from build123d import *

# Parameters (mm, degrees)
SKETCH1_W           = 15.24
SKETCH1_H           = 15.24
BOSS_EXTRUDE1_DEPTH = 25.146
SKETCH2_R           = 5.969
CUT_EXTRUDE1_DEPTH  = 22.4536
FILLET1_R           = 7.62
CUT_EXTRUDE2_DEPTH  = 22.4536
SKETCH4_R           = 1.4605
CUT_EXTRUDE3_DEPTH  = 32.123614073
SKETCH6_W           = 16.374741922
SKETCH6_H           = 17.109502327
CUT_EXTRUDE5_DEPTH  = 20.32
SKETCH5_W           = 2.54
SKETCH5_H           = 2.54
CUT_EXTRUDE4_DEPTH  = 6.35


with BuildPart() as part:
    # Sketch1 → Boss-Extrude1 (new body)
    with BuildSketch(Plane.XY):
        with Locations((7.62, 7.62)):
            Rectangle(SKETCH1_W, SKETCH1_H)
    extrude(amount=BOSS_EXTRUDE1_DEPTH)

    # Sketch2 → Cut-Extrude1 (cut)
    with BuildSketch(Plane.XY.offset(25.146)):
        with Locations((7.62, 7.62)):
            Circle(SKETCH2_R)
    extrude(amount=-CUT_EXTRUDE1_DEPTH, mode=Mode.SUBTRACT)

    # Fillet1
    fillet1_edges = [part.edges().sort_by_distance(p)[0] for p in [
        (15.24, 15.24, 12.573),
        (0, 15.24, 12.573),
    ]]
    fillet(fillet1_edges, radius=FILLET1_R - 0.0001)  # a hair under: the kernel refuses the full size

    # Sketch3 → Cut-Extrude2 (cut)
    with BuildSketch(Plane.XY.offset(25.146)):
        with BuildLine():
            Line((11.085783791, 12.479763751), (11.085783791, 15.600426387))
            Line((11.085783791, 15.600426387), (4.154216209, 15.600426387))
            Line((4.154216209, 15.600426387), (4.154216209, 12.479763751))
            ThreePointArc((4.154216209, 12.479763751), (7.62, 13.589), (11.085783791, 12.479763751))
        make_face()
    extrude(amount=-CUT_EXTRUDE2_DEPTH, mode=Mode.SUBTRACT)

    # Sketch4 → Cut-Extrude3 (cut, through all)
    with BuildSketch(Plane.XY.offset(2.6924)):
        with Locations((7.62, 7.62)):
            Circle(SKETCH4_R)
    extrude(amount=-CUT_EXTRUDE3_DEPTH, mode=Mode.SUBTRACT)

    # Sketch6 → Cut-Extrude5 (cut)
    with BuildSketch(Plane.XY.offset(25.146)):
        with Locations((8.187370961, 8.554751164)):
            Rectangle(SKETCH6_W, SKETCH6_H)
    extrude(amount=-CUT_EXTRUDE5_DEPTH, mode=Mode.SUBTRACT)

    # Sketch5 → Cut-Extrude4 (cut)
    with BuildSketch(Plane.XY.offset(25.146)):
        with Locations((1.27, 1.27)):
            Rectangle(SKETCH5_W, SKETCH5_H)
        with Locations((13.97, 1.27)):
            Rectangle(SKETCH5_W, SKETCH5_H)
    extrude(amount=-CUT_EXTRUDE4_DEPTH, mode=Mode.SUBTRACT)


solid = part.part
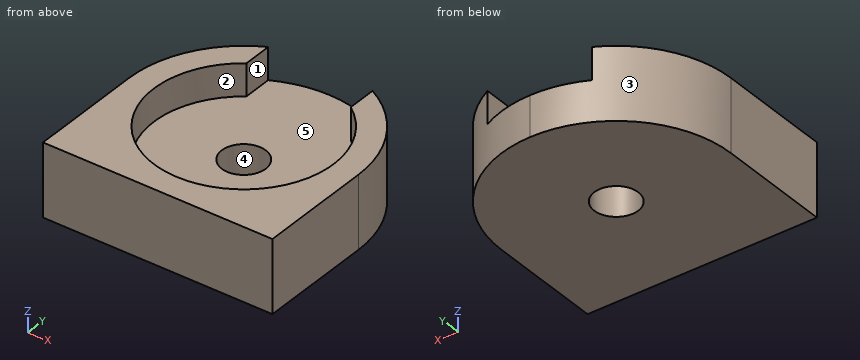
Part model, mm, in its own coordinate system. Face numbers are marked on the shaded views. A direction names the side the tool comes from. Give positions to 0.01 mm unless a question says otherwise; leave off trailing zeros. Loops run counter-clockwise (first coordinate to the right, second up) from the corner with the lowest first, then second, coordinate; pieces in that order, holes last. Notation, with made-up numbers: M -30,32.25 L 16,32.25 A15 cw 16,47.25 Z; hole C -40,26 d2. An arc over 180 degrees is marked long. Put each result on its own line as item: value. Start each with the question number.
1) Saw through at C-C (z = 3.45). List the corners of the cut face in (x, y).
2) Saw through at D-D (y = 12.75). List the corners of the cut face in (x, z).
3) Probe probe 1 along Y at (x, z) = (7.62, 1.5); probe 2 along X at (y, z) = (7.62, 4.3); probe 3 along Y at (x, z) = (7.62, 3.25). List the from-to ranges inside material, lowest first.
4) Pull direction Y, two halves, no side cores. Call the marked faces 1, 2 and 3: +Y half, -Y half, draft (parallel to the pull), parting line (faces both ways), or undercut.
5) 3-axis set-ups, long thin cutter, end or side, ignore diameter. For the marked faces 4 and 5: which of +Z, -Z, +X, -X, +Y, -Y reach the whole face in a straight line?
6) Saw through at B-B (y = 6.75). List the corners of the cut face in (x, z), then the cut area to 3 significant figures.
7) Flat gauge pins, fed straight in: pin 1 (3.5 mm diameter, centred on x = 6, y = 5.5, fed in from +Z); pin 2 (1 mm diameter, centred on y = 8.5, z = 2, fed in from +X); pin 3 (2 mm diameter, centred on x = 4.5, y = 12, fed in from -Z); pin 4 (1 mm diameter, centred on y = 13, z = 4, fed in from +X). Where does each tip first touch, or does it go through?
Numbers:
1. outline: M 0,0 L 15.24,0 L 15.24,7.62 A7.62 ccw 11.09,14.41 L 11.09,12.48 A5.97 cw long 4.15,12.48 L 4.15,14.41 A7.62 ccw 0,7.62 Z
2. outline: M 1.99,0 L 13.25,0 L 13.25,4.83 L 11.09,4.83 L 11.09,2.69 L 4.15,2.69 L 4.15,4.83 L 1.99,4.83 Z
3. probe 1: 0 to 6.16, 9.08 to 15.24
3. probe 2: 0 to 1.65, 13.59 to 15.24
3. probe 3: 0 to 1.65
4. face 1: draft
4. face 2: undercut
4. face 3: +Y half
5. face 4: +Z, -Z
5. face 5: +Z
6. outline: M 0,0 L 6.45,0 L 6.45,2.69 L 1.71,2.69 L 1.71,4.83 L 0,4.83 Z; M 8.79,0 L 15.24,0 L 15.24,4.83 L 13.53,4.83 L 13.53,2.69 L 8.79,2.69 Z
6. area: 42.0 mm^2
7. pin 1: z = 2.69
7. pin 2: x = 15.23
7. pin 3: z = 0
7. pin 4: x = 13.47
